Design review of the part built by this model. Coordinates are the model's own, in mm. Face numbers are marked on the shaded views. A direction names the side the tool comes from. Coordinates: 2 decimals unless noted, no trailing zeros. Loops run counter-clockwise (first coordinate to the right, second up) from the corner with the lowest first, then second, coordinate; pieces in that order, holes last. Notation, with made-up numbers: (-12.75, -22.5) -> (29.25, -22.5) arc R24 ccw to (29.25, 2.5) -> close; hole circle Ø9 at (39, -36). An arc over 180 degrees is marked (long way). Answer as a JSON object with one key per item and string values.
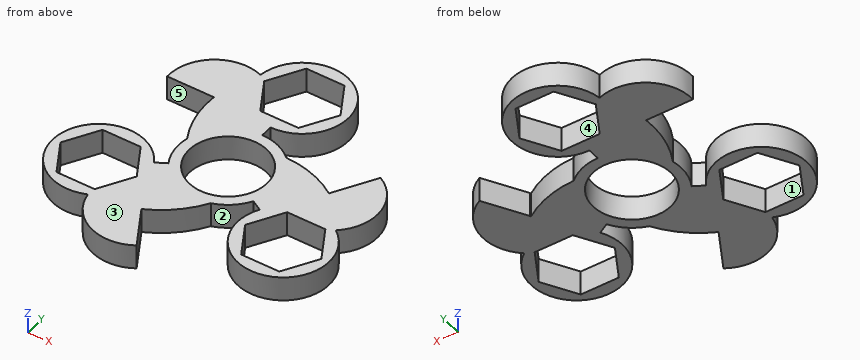
```python
from build123d import *

# Parameters (mm, degrees)
F0_R     = 11
F1_DEPTH = 7
F3_DEPTH = 25


with BuildPart() as f1:
    # F0 (on Top) → F1 (new body)
    with BuildSketch(Plane.XY):
        with BuildLine():
            ThreePointArc((-7.74528, -24.322292), (-0.888747, -19.704747), (4.347186, -13.307967))
            ThreePointArc((4.347186, -13.307967), (8.819044, -10.873108), (12.124356, -7))
            Line((12.124356, -7), (15.057621, -8.693521))
            ThreePointArc((15.057621, -8.693521), (28.99745, -27.91396), (33.992432, -4.702018))
            ThreePointArc((33.992432, -4.702018), (38.625506, 6.792291), (31.605888, 17.005492))
            Line((31.605888, 17.005492), (25.062695, 5.67235))
            Line((25.062695, 5.67235), (25.062695, 5.366495))
            ThreePointArc((25.062695, 5.366495), (17.582241, 9.059312), (9.351444, 10.418756))
            ThreePointArc((9.351444, 10.418756), (5.006866, 13.07407), (0, 14))
            Line((0, 14), (0, 17.387043))
            ThreePointArc((0, 17.387043), (9.675474, 39.069509), (-12.924149, 31.789318))
            ThreePointArc((-12.924149, 31.789318), (-25.19505, 30.054524), (-30.530132, 18.868756))
            Line((-30.530132, 18.868756), (-17.443746, 18.868756))
            Line((-17.443746, 18.868756), (-17.191083, 18.868756))
            ThreePointArc((-17.191083, 18.868756), (-16.620438, 10.62205), (-13.69863, 2.88921))
            ThreePointArc((-13.69863, 2.88921), (-13.825909, -2.200962), (-12.124356, -7))
            Line((-12.124356, -7), (-15.057621, -8.693521))
            ThreePointArc((-15.057621, -8.693521), (-38.672924, -11.155548), (-21.068283, -27.0873))
            ThreePointArc((-21.068283, -27.0873), (-13.430456, -36.846815), (-1.075755, -35.874248))
            Line((-1.075755, -35.874248), (-7.618949, -24.541105))
            Line((-7.618949, -24.541105), (-7.74528, -24.322292))
        make_face()
        Circle(F0_R, mode=Mode.SUBTRACT)
    extrude(amount=F1_DEPTH)

    # F2 (on face) → F3 (cut)
    with BuildSketch(Plane.XY.offset(7)):
        Polygon((5.435753, 39.802043), (-5.435753, 39.802043), (-10.871506, 30.387043), (-5.435753, 20.972043), (5.435753, 20.972043), (10.871506, 30.387043), align=None)
        Polygon((-37.187457, -15.193521), (-31.751704, -24.608521), (-20.880198, -24.608521), (-15.444446, -15.193521), (-20.880198, -5.778521), (-31.751704, -5.778521), align=None)
        Polygon((31.751704, -24.608521), (37.187457, -15.193521), (31.751704, -5.778521), (20.880198, -5.778521), (15.444446, -15.193521), (20.880198, -24.608521), align=None)
    extrude(amount=-F3_DEPTH, mode=Mode.SUBTRACT)


solid = f1.part
```
1) For the marked faces 1, 2 and 3, list the 3-axis set-ups (+Z, -Z, +X, -X, +Y, -Y) from which the entire face can be reached by the end or side of a thin tool; tool diameter is ignored.
Completed:
{"face 1": "+Z, -Z", "face 2": "+Z, -Z, -Y", "face 3": "+Z, +X, -X, +Y, -Y"}
2) Add section A-A, the plane x = -26. Give the boundary of the cut face in (y, z).
Completed:
{"outline": "(-28.19, 0) -> (-24.61, 0) -> (-24.61, 7) -> (-28.19, 7) -> close; (-5.78, 0) -> (-2.2, 0) -> (-2.2, 7) -> (-5.78, 7) -> close; (18.87, 0) -> (29.41, 0) -> (29.41, 7) -> (18.87, 7) -> close"}
3) Add section B-B, the plane y = 36.5. Give the boundary of the cut face in (x, z), and give its area (3 significant figures).
Completed:
{"outline": "(-11.47, 0) -> (-7.34, 0) -> (-7.34, 7) -> (-11.47, 7) -> close; (7.34, 0) -> (11.47, 0) -> (11.47, 7) -> (7.34, 7) -> close", "area": "57.8 mm²"}
4) Add section D-D, the plane z = 1.75. Count the separate pieces of the cut face and the enclosed holes in it, and give its area (3 significant figures).
Completed:
{"separate pieces": "1", "enclosed holes": "4", "area": "2,010 mm²"}
5) Clearance check with flat-ended pins moving along their axes: pin 1 Ø3 at (x, z) = (17.5, 5) entering from -Y; pin 2 Ø2 at (x, y) = (6.5, 5.5) entering from -Z; pin 3 Ø2 at (x, z) = (-23, 3) entering from -Y; pin 4 Ø2 at (x, z) = (-2, 1) entering from +Y. State where each tip first meets the part, or that it passes through.
Completed:
{"pin 1": "y = -25.94", "pin 2": "through", "pin 3": "y = -27.99", "pin 4": "y = 43.35"}
6) Wall thickness on probe 1 along Y at (x, z) = (-26.5, 2.5); probe 2 along Y at (x, z) = (-28, 4.5); probe 3 along Y at (x, z) = (32, 1): over which ranges is each line inside the solid? List them lowest first.
Completed:
{"probe 1": "-28.19 to -24.61, -5.78 to -2.19, 18.87 to 28.96", "probe 2": "-28.08 to -24.61, -5.78 to -2.3, 18.87 to 27.25", "probe 3": "-26.89 to -24.18, -6.21 to 16.79"}
7) The part is to be moulded in two halves that separate along X. For the marked faces 4 and 5, say which applies: pulls with the +X half, pulls with the -X half, needs draft (parallel to the pull), parting line crosses it, or undercut.
Completed:
{"face 4": "undercut", "face 5": "needs draft"}
8) Add section C-C, the plane x = 18.5. Give the boundary of the cut face in (y, z).
Completed:
{"outline": "(-25.58, 0) -> (-20.49, 0) -> (-20.49, 7) -> (-25.58, 7) -> close; (-9.9, 0) -> (8.75, 0) -> (8.75, 7) -> (-9.9, 7) -> close"}
